Work out the finished part from the listing and answer in its coordinate system (mm). A direction names the side the tool comes from. Give positions to 0.01 mm unless a question says otherwise; leave off trailing zeros. Loops run counter-clockwise (first coordinate to the right, second up) from the corner with the lowest first, then second, coordinate; pieces in that order, holes last. Notation, with made-up numbers: (-13, -36.75) -> (14, -36.75) arc R6 ccw to (14, -26.75) -> close; hole circle Ø3 at (32.5, 86.5). An arc over 180 degrees is marked (long way). Answer as CSV lines item,"result". Start each with the question number.
1. Determine the mould class of faces 1 (the face through (-5.54, 12.78, 16.18)), 2 (the face through (27, 15, 20)), 3 (the face through (-25, 27, 11)), 4 (the face through (6.81, 11.5, 26.86)) for opening direction X: +X half, -X half, draft (parallel to the pull), parting line (faces both ways), or undercut.
2. Find section A-A, the plane x = 0. Give the vertices of the cut face in (y, z) (3 decimals), and give its area (3 significant figures).
3. Find section C-C, the plane y = 5. Give the vertices of the cut face in (x, z).
4. Find the intervals of material crossed by line 1 along X through (y, z) = (12.5, 24.5); line 2 along Y through (x, z) = (-5.5, 24.25); line 3 along Y through (x, z) = (5.5, 22), in increasing order.
5. Flat-ended cylindrical pins translate along their axes: pin 1 Ø4 at (x, y) = (21.5, 30.5) entering from +Z; pin 2 Ø12.5 at (y, z) = (29.5, 24.5) entering from +X; pin 3 Ø1.5 at (x, z) = (-26.5, 13.5) entering from +Y; pin 4 Ø4 at (x, y) = (5.5, 12.5) entering from +Z. Find the tip coordinate at first contact, or state that the pin passes through.
6. Find section D-D, the plane z = 9. Give the vertices of the cut face in (x, y), and give its area (3 significant figures).
7. Find section B-B, the plane z = 29. Give the vertices of the cut face in (x, y), and give its area (3 significant figures).
8. A tool of negligible diameter and unlimited length cuts with its end or side. For faces 5 (the face through (-28, 15, 20)), 6 (the face through (-11, 9, 39)), 7 (the face through (0, 32, 5)), 8 (the face through (0, 17.5, 34)), 9 (the face through (25, 27, 11)), from which of +Z, -Z, +X, -X, +Y, -Y can it reach the whole face along a straight path? Write none if from no direction.
from build123d import *

# Parameters (mm, degrees)
F0_W            = 60
F0_H            = 40
F1_DEPTH        = 40
F2_W            = 5
F2_H            = 25
F3_DEPTH        = 40.001
F5_DEPTH        = 55.001
F7_DEPTH        = 40.001
F8_W            = 22
F8_H            = 17.5
F9_DEPTH        = 3
F11_D           = 3.3
F11_DEPTH       = 20
F11_TIP         = 0.9914200214
F13_D           = 8.8
F13_DEPTH       = 50
F13_CBORE_D     = 14.25
F13_CBORE_DEPTH = 8
F13_TIP         = 2.6437867237


with BuildPart() as f1:
    # F0 (on Top) → F1 (new body)
    with BuildSketch(Plane.XY):
        with Locations((0, 20)):
            Rectangle(F0_W, F0_H)
    extrude(amount=F1_DEPTH)

    # F2 (on face) → F3 (cut, through all)
    with BuildSketch(Plane.XY.offset(40)):
        with Locations((-27.5, 27.5)):
            Rectangle(F2_W, F2_H)
        with Locations((27.5, 27.5)):
            Rectangle(F2_W, F2_H)
    extrude(amount=-F3_DEPTH, mode=Mode.SUBTRACT)

    # F4 (on face) → F5 (cut, through all)
    with BuildSketch(Plane.YZ.offset(25)):
        with BuildLine():
            ThreePointArc((17.5, 27), (27.5, 17), (37.5, 27))
            ThreePointArc((37.5, 27), (27.5, 37), (17.5, 27))
        make_face()
        with BuildLine():
            ThreePointArc((17.5, 27), (27.5, 37), (37.5, 27))
            Line((37.5, 27), (40, 27))
            Line((40, 27), (40, 40))
            Line((40, 40), (17.5, 40))
            Line((17.5, 40), (17.5, 27))
        make_face()
    extrude(amount=-F5_DEPTH, mode=Mode.SUBTRACT)

    # F6 (on face) → F7 (cut, through all)
    with BuildSketch(Plane.XY.offset(40)):
        with BuildLine():
            Line((-24, 0), (-16, 0))
            ThreePointArc((-16, 0), (-20, 4), (-24, 0))
        make_face()
        with BuildLine():
            ThreePointArc((24, 0), (20, 4), (16, 0))
            Line((16, 0), (24, 0))
        make_face()
    extrude(amount=-F7_DEPTH, mode=Mode.SUBTRACT)

    # F8 (on face) → F9 (cut)
    with BuildSketch(Plane.XY.offset(40)):
        with Locations((0, 8.75)):
            Rectangle(F8_W, F8_H)
    extrude(amount=-F9_DEPTH, mode=Mode.SUBTRACT)

    # F11
    with Locations(Plane.XY.offset(37)):
        with Locations((-5.5, 12.5), (5.5, 12.5)):
            Hole(F11_D / 2, depth=F11_DEPTH)
            with Locations((0, 0, -(F11_DEPTH + F11_TIP / 2))):  # 118° drill point
                Cone(0, F11_D / 2, F11_TIP, mode=Mode.SUBTRACT)

    # F13
    with Locations(Plane(origin=(0, 40, 0), x_dir=(-1, 0, 0), z_dir=(0, 1, 0))):
        with Locations((0, 10)):
            CounterBoreHole(F13_D / 2, F13_CBORE_D / 2, F13_CBORE_DEPTH, depth=F13_DEPTH)
            with Locations((0, 0, -(F13_DEPTH + F13_TIP / 2))):  # 118° drill point
                Cone(0, F13_D / 2, F13_TIP, mode=Mode.SUBTRACT)


solid = f1.part
Resolved:
1,face 1,"undercut"
1,face 2,"draft"
1,face 3,"-X half"
1,face 4,"undercut"
2,outline,"(0, 0) -> (40, 0) -> (40, 2.875) -> (32, 2.875) -> (32, 5.6) -> (0, 5.6) -> close; (0, 14.4) -> (32, 14.4) -> (32, 17.125) -> (40, 17.125) -> (40, 27) -> (37.5, 27) arc R10 cw to (17.5, 27) -> (17.5, 37) -> (0, 37) -> close"
2,area,"702 mm^2"
3,outline,"(-30, 0) -> (30, 0) -> (30, 40) -> (11, 40) -> (11, 37) -> (-11, 37) -> (-11, 40) -> (-30, 40) -> close; hole circle Ø8.8 at (0, 10)"
4,line 1,"x = -30 to -7.15, -3.85 to 3.85, 7.15 to 30"
4,line 2,"y = 0 to 10.85, 14.15 to 17.89, 37.11 to 40"
4,line 3,"y = 0 to 10.85, 14.15 to 18.84, 36.16 to 40"
5,pin 1,"stops at z = 18.34"
5,pin 2,"passes through"
5,pin 3,"stops at y = 15"
5,pin 4,"stops at z = 37"
6,outline,"(-30, 0) -> (-24, 0) arc R4 cw to (-16, 0) -> (-4.28, 0) -> (-4.28, 32) -> (-7.05, 32) -> (-7.05, 40) -> (-25, 40) -> (-25, 15) -> (-30, 15) -> close; (4.28, 0) -> (16, 0) arc R4 cw to (24, 0) -> (30, 0) -> (30, 15) -> (25, 15) -> (25, 40) -> (7.05, 40) -> (7.05, 32) -> (4.28, 32) -> close"
6,area,"1,710 mm^2"
7,outline,"(-30, 0) -> (-24, 0) arc R4 cw to (-16, 0) -> (16, 0) arc R4 cw to (24, 0) -> (30, 0) -> (30, 15) -> (25, 15) -> (25, 17.5) -> (-25, 17.5) -> (-25, 15) -> (-30, 15) -> close; hole circle Ø3.3 at (-5.5, 12.5); hole circle Ø3.3 at (5.5, 12.5)"
7,area,"958 mm^2"
8,face 5,"+Z, -Z, -X, +Y"
8,face 6,"+Z, +Y, -Y"
8,face 7,"+Y"
8,face 8,"+Z, +X, -X, +Y"
8,face 9,"+Z, -Z, +X, +Y"
